Part model, mm, in its own coordinate system. A direction names the side the tool comes from. Coordinates: 2 decimals unless noted, no trailing zeros. Loops run counter-clockwise (first coordinate to the right, second up) from the corner with the lowest first, then second, coordinate; pieces in that order, holes last.
```python
from build123d import *

# Parameters (mm, degrees)
SKETCH_3_R          = 17.5
SKETCH_3_R_2        = 4
EXTRUDE_1_DEPTH     = 10
CUT_EXTRUDE_1_DEPTH = 0.5


with BuildPart() as part:
    # 草图3 → 凸台-拉伸1 (new body)
    with BuildSketch(Plane(origin=(0, 0, 0), x_dir=(1, 0, 0), z_dir=(0, 1, 0))):
        with Locations(Location((-175, 0, 0), (0, 0, 270))):
            Circle(SKETCH_3_R)
        with Locations(Location((-175, 0, 0), (0, 0, 270))):
            Circle(SKETCH_3_R_2, mode=Mode.SUBTRACT)
    extrude(amount=EXTRUDE_1_DEPTH)

    # 草图5 → 切除-拉伸1 (cut)
    with BuildSketch(Plane(origin=(0, 10, 0), x_dir=(1, 0, 0), z_dir=(0, 1, 0))):
        with BuildLine():
            ThreePointArc((-164.451502199, -12.878997225), (-158.353020286, 0.132067312), (-164.657165804, 13.044736723))
            ThreePointArc((-164.657165804, 13.044736723), (-166.97169342, 12.777345636), (-166.704302333, 10.46281802))
            ThreePointArc((-166.704302333, 10.46281802), (-161.647923755, 0.105927492), (-166.539345315, -10.32988301))
            ThreePointArc((-166.539345315, -10.32988301), (-166.769980864, -12.648361675), (-164.451502199, -12.878997225))
        make_face()
        with BuildLine():
            ThreePointArc((-185.548497801, -12.878997225), (-191.646979714, 0.132067312), (-185.342834196, 13.044736723))
            ThreePointArc((-185.342834196, 13.044736723), (-183.02830658, 12.777345636), (-183.295697667, 10.46281802))
            ThreePointArc((-183.295697667, 10.46281802), (-188.352076245, 0.105927492), (-183.460654685, -10.32988301))
            ThreePointArc((-183.460654685, -10.32988301), (-183.230019136, -12.648361675), (-185.548497801, -12.878997225))
        make_face()
    extrude(amount=-CUT_EXTRUDE_1_DEPTH, mode=Mode.SUBTRACT)


solid = part.part
```
Q1. Saw through at A-A (x = -175). List the corners of the cut face in (y, z).
Q2. Drop flat-ended pins along their axis: P1, Ø6, axis at x = -182.5, y = 5.5, coming from the -Z side; P2, Ø4, axis at y = 4, z = -12.5, coming from the -X side; P3, Ø4, axis at y = 4, z = -11.5, coming from the +X side. Give the stop position or say it passes through.
Q3. Probe line 1 (X direction, y = 7, z = 0); line 2 (Z direction, x = -176, y = 0.5); line 3 (Z direction, x = -176.5, y = 2.5). List the from-to ranges inside material, lowest first.
Q4. Saw through at B-B (z = 0). List the corners of the cut face in (x, y), plus the area to 3 significant figures.
Q5. Saw through at C-C (z = 7). List the corners of the cut face in (x, y).
Q6. Saw through at D-D (x = -160.5). List the corners of the cut face in (y, z), plus the area to 3 significant figures.
Q7. Tool access for faces 4 (the flat face through (-179, 10, 4)), 5 (the cylindrical face through (-183.207, 9.754, 12.62)): list every direction of +Z, -Z, +X, -X, +Y, -Y with a clear straight run to the whole face (end or side of a thin tool).
Q8. Mould opens along Z. For faces 1 (the cylindrical face through (-157.65, 4.93, -2.28)), 2 (the cylindrical face through (-183.051, 9.754, -12.805)), 3 (the flat face through (-179, 0, 4)) say: released by +Z, released by -Z, zero draft, split by the parting line, or undercut.
Checked values:
1. outline: (0, -17.5) - (10, -17.5) - (10, -4) - (0, -4) - close; (0, 4) - (10, 4) - (10, 17.5) - (0, 17.5) - close
2. P1: stops at z = -16.91
2. P2: stops at x = -189
2. P3: stops at x = -160.3
3. line 1: x = -192.5 to -179, -171 to -157.5
3. line 2: z = -17.47 to -3.87, 3.87 to 17.47
3. line 3: z = -17.44 to -3.71, 3.71 to 17.44
4. outline: (-192.5, 0) - (-179, 0) - (-179, 10) - (-188.35, 10) - (-188.35, 9.5) - (-191.65, 9.5) - (-191.65, 10) - (-192.5, 10) - close; (-171, 0) - (-157.5, 0) - (-157.5, 10) - (-158.35, 10) - (-158.35, 9.5) - (-161.65, 9.5) - (-161.65, 10) - (-171, 10) - close
4. area: 267 mm2
5. outline: (-191.04, 0) - (-158.96, 0) - (-158.96, 10) - (-159.9, 10) - (-159.9, 9.5) - (-163.63, 9.5) - (-163.63, 10) - (-186.37, 10) - (-186.37, 9.5) - (-190.1, 9.5) - (-190.1, 10) - (-191.04, 10) - close
6. outline: (0, -9.8) - (10, -9.8) - (10, -8.18) - (9.5, -8.18) - (9.5, 8.18) - (10, 8.18) - (10, 9.8) - (0, 9.8) - close
6. area: 188 mm2
7. face 4: +Z, -Z, +X, -X, +Y
7. face 5: +Y
8. face 1: split by the parting line
8. face 2: undercut
8. face 3: zero draft
